For this review, use the dimensioned drawing (mm, ordinates from the lowest corner) and the shaded views. A direction names the side the tool comes from. Round coordinates to 2 decimals unless told otherwise and drop trailing zeros. Loops run counter-clockwise (first coordinate to the right, second up) from the corner with the lowest first, then second, coordinate; pieces in that order, holes last. Notation, with made-up numbers: (-36, 32) -> (-13, 32) arc R20 ccw to (-13, 59) -> close; hole circle Ø7 at (-32.75, 17.25). An arc over 180 degrees is marked (long way). Use one line per item in the form item = value. Start each with the question number.
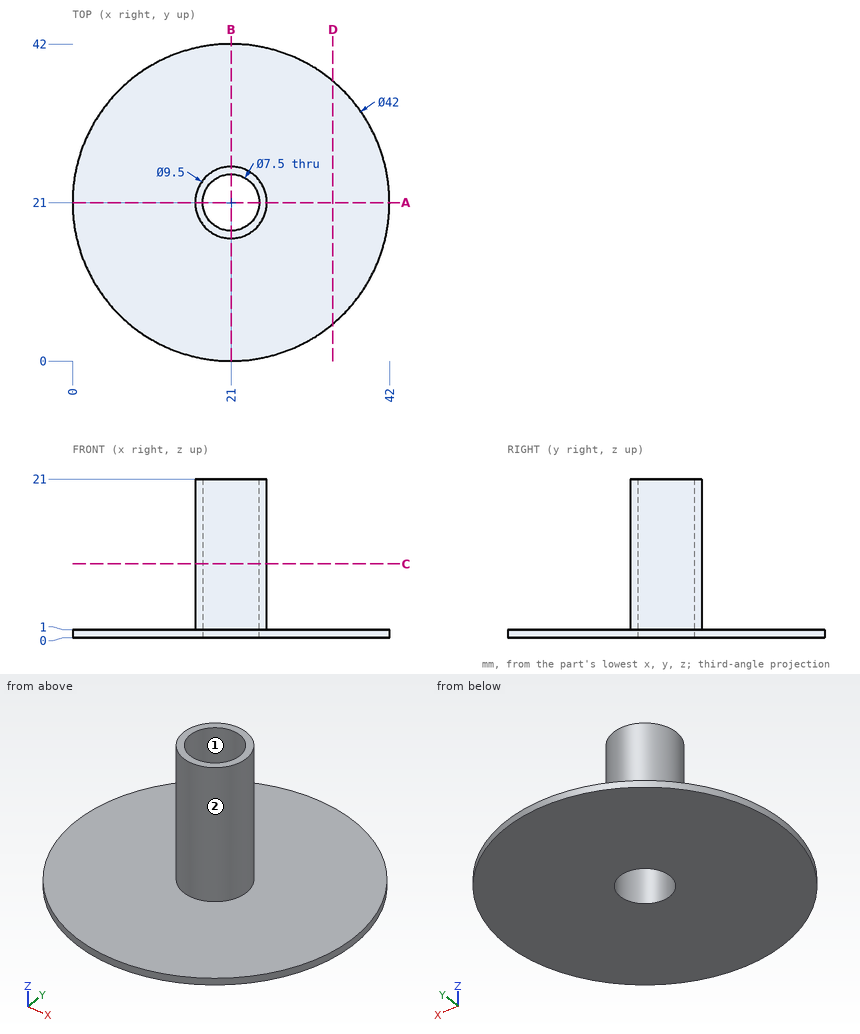
Item 1: Take a section at D-D on x = 34.5. Give the boundary of the cut face in (y, z).
Item 2: Take a section at C-C on z = 9.75. Give the boundary of the cut face in (x, y), plus the area to 3 significant figures.
Item 3: Take a section at A-A on y = 21. Give the boundary of the cut face in (x, z), plus the area to 3 significant figures.
Item 4: Wall thickness on line 1 (Y direction, x = 21, z = 19.25); line 2 (Z direction, x = 9, y = 15.5); line 3 (X direction, y = 23.5, z = 6): over which ranges is each line inside the solid? List them lowest first.
Item 5: For P1, Ø3, axis at x = 10, y = 25, coming from the +Z side; P2, Ø12, axis at y = 9, z = 13.5, coming from the +X side; P3, Ø2, axis at x = 24, z = 11.5, coming from the +Y side; P4, Ø8, axis at y = 21, z = 16.5, coming from the -X side, all flat-tipped, find the tip position at first contact; note any pin that passes through.
Item 6: Machinability: for the marked faces 1 and 2, which of the approach directions +Z, -Z, +X, -X, +Y, -Y give a long, thin tool a straight path to every point of the face, cutting with its end or side? Answer none if there is none.
Results:
q1.outline = (4.91, 0) -> (37.09, 0) -> (37.09, 1) -> (4.91, 1) -> close
q2.outline = circle Ø9.5 at (21, 21); hole circle Ø7.5 at (21, 21)
q2.area = 26.7 mm2
q3.outline = (0, 0) -> (17.25, 0) -> (17.25, 21) -> (16.25, 21) -> (16.25, 1) -> (0, 1) -> close; (24.75, 0) -> (42, 0) -> (42, 1) -> (25.75, 1) -> (25.75, 21) -> (24.75, 21) -> close
q3.area = 74.5 mm2
q4.line_1 = 16.25 to 17.25, 24.75 to 25.75
q4.line_2 = 0 to 1
q4.line_3 = 16.96 to 18.2, 23.8 to 25.04
q5.P1 = 1
q5.P2 = through
q5.P3 = 25.31
q5.P4 = 16.25
q6.face_1 = +Z, -Z
q6.face_2 = +Z
